from build123d import *

# Parameters (mm, degrees)
BOSS_EXTRUDE2_DEPTH = 6.35
CUT_EXTRUDE1_REACH  = 129.376
SKETCH4_W           = 12.7
SKETCH4_H           = 12.7


with BuildPart() as part:
    # Sketch3 → Boss-Extrude2 (new body)
    with BuildSketch(Plane(origin=(0, 0, 0), x_dir=(0, 0, -1), z_dir=(1, 0, 0))):
        with BuildLine():
            Line((-57.15, -110.236), (57.15, -110.236))
            ThreePointArc((57.15, -110.236), (61.640128061, -108.376128061), (63.5, -103.886))
            Line((63.5, -103.886), (63.5, 103.886))
            ThreePointArc((63.5, 103.886), (61.640128061, 108.376128061), (57.15, 110.236))
            Line((57.15, 110.236), (-57.15, 110.236))
            ThreePointArc((-57.15, 110.236), (-61.640128061, 108.376128061), (-63.5, 103.886))
            Line((-63.5, 103.886), (-63.5, -103.886))
            ThreePointArc((-63.5, -103.886), (-61.640128061, -108.376128061), (-57.15, -110.236))
        make_face()
        with BuildLine():
            Line((-31.75, -67.564), (31.75, -67.564))
            ThreePointArc((31.75, -67.564), (36.240128061, -65.704128061), (38.1, -61.214))
            Line((38.1, -61.214), (38.1, 78.486))
            ThreePointArc((38.1, 78.486), (36.240128061, 82.976128061), (31.75, 84.836))
            Line((31.75, 84.836), (-31.75, 84.836))
            ThreePointArc((-31.75, 84.836), (-36.240128061, 82.976128061), (-38.1, 78.486))
            Line((-38.1, 78.486), (-38.1, -61.214))
            ThreePointArc((-38.1, -61.214), (-36.240128061, -65.704128061), (-31.75, -67.564))
        make_face(mode=Mode.SUBTRACT)
    extrude(amount=BOSS_EXTRUDE2_DEPTH)

    # Sketch4 → Cut-Extrude1 (cut, up to next)
    with BuildSketch(Plane(origin=(6.35, 0, 0), x_dir=(0, 0, -1), z_dir=(1, 0, 0)), mode=Mode.PRIVATE) as cut_extrude1_sk1:
        with Locations((0, -91.186)):
            Rectangle(SKETCH4_W, SKETCH4_H)
    cut_extrude1_tool1 = extrude(cut_extrude1_sk1.sketch, amount=-CUT_EXTRUDE1_REACH, mode=Mode.PRIVATE) & part.part
    add(cut_extrude1_tool1.solids().sort_by_distance((6.35, -91.186, 0))[0], mode=Mode.SUBTRACT)


solid = part.part
The model under review builds one solid part; all positions refer to its coordinate system, in mm. A direction names the side the tool comes from. Give positions to 0.01 mm unless a question says otherwise; leave off trailing zeros. Write each loop counter-clockwise with the first axis right and the second up, starting at its lowest first coordinate (ties: lowest second). Pieces come first, ordered by that corner, then holes.
1. Add section A-A, the plane z = -21.5. Write out the cut boundary in (x, y).
2. Add section B-B, the plane y = 58. Write out the cut boundary in (x, z), plus the area to 3 significant figures.
3. Add section D-D, the plane z = -3. Write out the cut boundary in (x, y), plus the area to 3 significant figures.
4. Wall thickness on L1, parallel to Z at x = 4, y = -7.5; L2, parallel to Y at x = 3.5, z = -8.5; L3, parallel to Z at x = 2.25, y = -96.5: over which ranges is each line inside the solid? List them lowest first.
5. Tool access review of faces 4 (the flat face through (3, -110.236, 1)), 5 (the flat face through (3, 84.836, 0)): name each direction out of +Z, -Z, +X, -X, +Y, -Y from which nothing blocks a thin tool from reaching the whole face with its end or side.
6. Add section C-C, the plane x = 1. Write out the cut boundary in (y, z).
7. Draft analysis for pull direction Y (two halves, no side actions). For faces 1 (the cylindrical face through (3.131, -108.425, -61.59)), 2 (the flat face through (0, 2, 43)), 3 (the flat face through (3, -67.564, 0)), state which applies: +Y half, -Y half, draft (parallel to the pull), parting line (faces both ways), or undercut.
Worked answers:
1. outline: (0, -110.24) - (6.35, -110.24) - (6.35, -67.56) - (0, -67.56) - close; (0, 84.84) - (6.35, 84.84) - (6.35, 110.24) - (0, 110.24) - close
2. outline: (0, -63.5) - (6.35, -63.5) - (6.35, -38.1) - (0, -38.1) - close; (0, 38.1) - (6.35, 38.1) - (6.35, 63.5) - (0, 63.5) - close
2. area: 323 mm2
3. outline: (0, -110.24) - (6.35, -110.24) - (6.35, -97.54) - (0, -97.54) - close; (0, -84.84) - (6.35, -84.84) - (6.35, -67.56) - (0, -67.56) - close; (0, 84.84) - (6.35, 84.84) - (6.35, 110.24) - (0, 110.24) - close
3. area: 352 mm2
4. L1: z = -63.5 to -38.1, 38.1 to 63.5
4. L2: y = -110.24 to -67.56, 84.84 to 110.24
4. L3: z = -63.5 to -6.35, 6.35 to 63.5
5. face 4: +Z, -Z, +X, -X, -Y
5. face 5: +X, -X
6. outline: (-110.24, -57.15) arc R6.35 ccw to (-103.89, -63.5) - (103.89, -63.5) arc R6.35 ccw to (110.24, -57.15) - (110.24, 57.15) arc R6.35 ccw to (103.89, 63.5) - (-103.89, 63.5) arc R6.35 ccw to (-110.24, 57.15) - close; hole (-97.54, -6.35) - (-84.84, -6.35) - (-84.84, 6.35) - (-97.54, 6.35) - close; hole (-67.56, -31.75) arc R6.35 ccw to (-61.21, -38.1) - (78.49, -38.1) arc R6.35 ccw to (84.84, -31.75) - (84.84, 31.75) arc R6.35 ccw to (78.49, 38.1) - (-61.21, 38.1) arc R6.35 ccw to (-67.56, 31.75) - close
7. face 1: -Y half
7. face 2: draft
7. face 3: undercut
